```python
from build123d import *

# Parameters (mm, degrees)
F1_DEPTH  = 426.72
F3_DEPTH  = 121.92
F5_DEPTH  = 304.8
F6_R      = 66.226706
F7_R      = 58.868184
F8_W      = 1436.773274
F8_H      = 347.196668
F9_DEPTH  = 15.24
F10_W     = 491.156265
F10_H     = 28.227374
F10_W_2   = 533.497333
F11_DEPTH = 9.144
F12_W     = 550.433874
F12_H     = 378.246805
F13_DEPTH = 381
F14_W     = 550.433874
F14_H     = 22.581905
F14_H_2   = 25.404632
F15_DEPTH = 381


with BuildPart() as f1:
    # F0 (on Top) → F1 (new body)
    with BuildSketch(Plane.XY):
        Polygon((2133.6, 0), (0, 0), (0, -609.6), (1524, -609.6), (1524, -1371.6), (2133.6, -1371.6), align=None)
    extrude(amount=F1_DEPTH)

    # F2 (on face) → F3 (join)
    with BuildSketch(Plane.XY.offset(426.72)):
        Polygon((2133.6, 0), (27.330885, 0), (27.330885, -566.014111), (1553.559542, -566.014111), (1553.559542, -1331.258059), (2133.6, -1331.258059), align=None)
    extrude(amount=F3_DEPTH)

    # F4 (on face) → F5 (join)
    with BuildSketch(Plane.XY.offset(548.64)):
        Polygon((2133.6, 0), (27.330885, 0), (27.330885, -152.4), (1981.2, -152.4), (1981.2, -1331.258059), (2133.6, -1331.258059), align=None)
    extrude(amount=F5_DEPTH)

    # F6
    f6_edges = [f1.edges().sort_by_distance(p)[0] for p in [
        (27.330885, -566.014111, 487.68),
        (1553.559542, -566.014111, 487.68),
        (1553.559542, -1331.258059, 487.68),
    ]]
    fillet(f6_edges, radius=F6_R)

    # F7
    f7_edges = [f1.edges().sort_by_distance(p)[0] for p in [
        (27.330885, -76.2, 853.44),
        (2057.4, -1331.258059, 853.44),
    ]]
    fillet(f7_edges, radius=F7_R)

    # F8 (on face) → F9 (join)
    with BuildSketch(Plane.XZ.offset(609.6)):
        with Locations((754.894508, 207.948759)):
            Rectangle(F8_W, F8_H)
    extrude(amount=F9_DEPTH)

    # F10 (on face) → F11 (join)
    with BuildSketch(Plane.XZ.offset(624.84)):
        with Locations((369.590856, 248.878457)):
            Rectangle(F10_W, F10_H)
        with Locations((963.777065, 248.878457)):
            Rectangle(F10_W_2, F10_H)
    extrude(amount=F11_DEPTH)

    # F12 (on face) → F13 (cut)
    with BuildSketch(Plane.XZ.offset(1371.6)):
        with Locations((1830.357432, 212.182869)):
            Rectangle(F12_W, F12_H)
    extrude(amount=-F13_DEPTH, mode=Mode.SUBTRACT)

    # F14 (on face) → F15 (join)
    with BuildSketch(Plane.XZ.offset(990.6)):
        with Locations((1830.357432, 285.574033)):
            Rectangle(F14_W, F14_H)
        with Locations((1830.357432, 162.784964)):
            Rectangle(F14_W, F14_H_2)
    extrude(amount=F15_DEPTH)


solid = f1.part
```
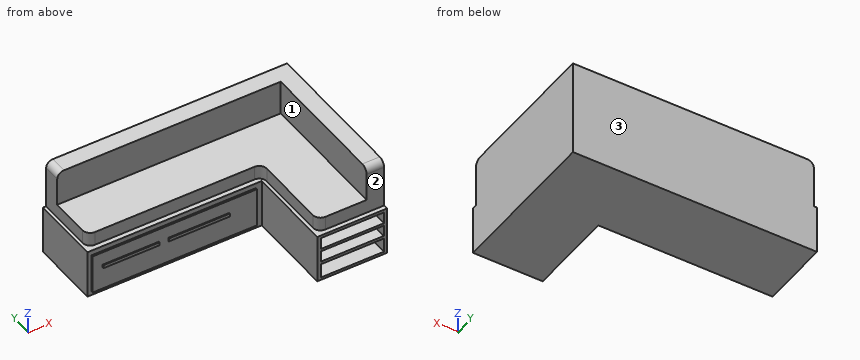
Part model, mm, in its own coordinate system. Face numbers are marked on the shaded views. A direction names the side the tool comes from. Give positions to 0.01 mm unless a question says otherwise; leave off trailing zeros. Write each loop counter-clockwise with the first axis right and the second up, starting at its lowest first coordinate (ties: lowest second). Pieces come first, ordered by that corner, then holes. Notation, with made-up numbers: (77, 10.5) -> (85, 10.5) arc R20 cw to (85, 45.5) -> close; hole circle Ø1 at (65, 23.5). An arc over 180 degrees is marked (long way). Put each result on its own line as item: value. Start each with the question number.
Item 1: Pin check, flat tips, straight feed: pin 1 Ø12 at (x, z) = (573.5, 530.5) entering from -Y; pin 2 Ø6 at (x, y) = (1855, -771.5) entering from +Z; pin 3 Ø8 at (x, z) = (1102.5, 447.5) entering from +Y; pin 4 Ø7.5 at (x, y) = (345, -627.5) entering from -Z. Stop position of each tip, or through.
Item 2: Cut at C-C (z = 106). List the corners of the cut face in (x, y), then the cut area to 3 significant figures.
Item 3: Cut at B-B (y = -1023). List the corners of the cut face in (x, z).
Item 4: Wall check: L1, parallel to Y at x = 1015, z = 600; L2, parallel to Z at x = 1567, y = -514; L3, parallel to Y at x = 1223.5, z = 125. Give the ranges that are in metal, low to high. Write a range as [from, to].
Item 5: Which spindle directions (+Z, -Z, +X, -X, +Y, -Y) get a long thin tool onto all of the face, cutting with end or side? Do the marked faces 1, 2 and 3. Say none if no direction does.
Item 6: Cut at A-A (x = 1767). List the corners of the cut face in (y, z).
Item 7: Cut at D-D (y = -260). List the corners of the cut face in (x, z).
Answer list:
1. pin 1: stops at y = -566.01
1. pin 2: stops at z = 548.64
1. pin 3: stops at y = 0
1. pin 4: stops at z = 34.35
2. outline: (0, -609.6) -> (36.51, -609.6) -> (36.51, -624.84) -> (1473.28, -624.84) -> (1473.28, -609.6) -> (1524, -609.6) -> (1524, -1371.6) -> (1555.14, -1371.6) -> (1555.14, -990.6) -> (2105.57, -990.6) -> (2105.57, -1371.6) -> (2133.6, -1371.6) -> (2133.6, 0) -> (0, 0) -> close
2. area: 1,580,000 mm2
3. outline: (1524, 0) -> (2133.6, 0) -> (2133.6, 853.44) -> (1981.2, 853.44) -> (1981.2, 548.64) -> (1553.56, 548.64) -> (1553.56, 426.72) -> (1524, 426.72) -> close; hole (1555.14, 23.06) -> (2105.57, 23.06) -> (2105.57, 150.08) -> (1555.14, 150.08) -> close; hole (1555.14, 175.49) -> (2105.57, 175.49) -> (2105.57, 274.28) -> (1555.14, 274.28) -> close; hole (1555.14, 296.86) -> (2105.57, 296.86) -> (2105.57, 401.31) -> (1555.14, 401.31) -> close
4. L1: y = [-152.4, 0]
4. L2: z = [0, 548.64]
4. L3: y = [-624.84, 0]
5. face 1: +Z, -X, -Y
5. face 2: +Z, +X, -X, -Y
5. face 3: +Z, -Z, +X, -X, +Y
6. outline: (-1371.6, 0) -> (0, 0) -> (0, 853.44) -> (-152.4, 853.44) -> (-152.4, 548.64) -> (-1331.26, 548.64) -> (-1331.26, 426.72) -> (-1371.6, 426.72) -> (-1371.6, 401.31) -> (-990.6, 401.31) -> (-990.6, 296.86) -> (-1371.6, 296.86) -> (-1371.6, 274.28) -> (-990.6, 274.28) -> (-990.6, 175.49) -> (-1371.6, 175.49) -> (-1371.6, 150.08) -> (-990.6, 150.08) -> (-990.6, 23.06) -> (-1371.6, 23.06) -> close
7. outline: (0, 0) -> (2133.6, 0) -> (2133.6, 853.44) -> (1981.2, 853.44) -> (1981.2, 548.64) -> (27.33, 548.64) -> (27.33, 426.72) -> (0, 426.72) -> close
